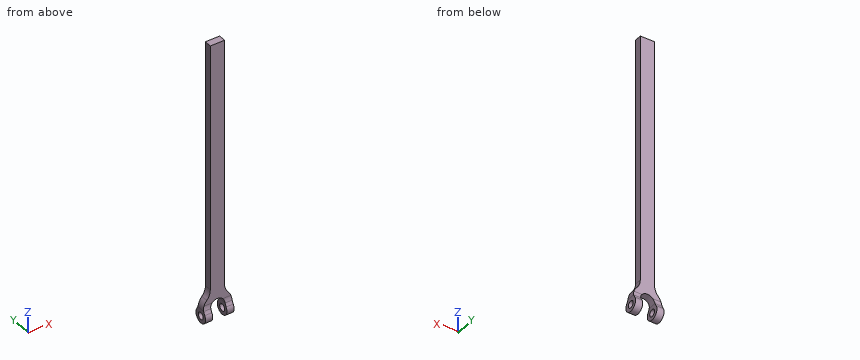
```python
from build123d import *

# Parameters (mm, degrees)
BOSS_EXTRUDE1_DEPTH = 10
CUT_EXTRUDE5_DEPTH  = 103.46950766


with BuildPart() as part:
    # Sketch1 → Boss-Extrude1 (new body)
    with BuildSketch(Plane(origin=(0, 0, 0), x_dir=(1, 0, 0), z_dir=(0, 1, 0))):
        with BuildLine():
            ThreePointArc((5, 90), (0, 85), (-5, 90))
            Line((-5, 90), (-5, 98.660254038))
            ThreePointArc((-5, 98.660254038), (-8.660254037, 95.000000002), (-10, 90.000000004))
            ThreePointArc((-10, 90.000000004), (-9.354143468, 86.464466096), (-7.5, 83.385621722))
            ThreePointArc((-7.5, 83.385621722), (-5.645856533, 80.306777351), (-5, 76.771243445))
            Line((-5, 76.771243445), (-5, -100))
            Line((-5, -100), (5, -100))
            Line((5, -100), (5, 76.771243445))
            ThreePointArc((5, 76.771243445), (5.645856533, 80.306777351), (7.5, 83.385621722))
            ThreePointArc((7.5, 83.385621722), (9.354143466, 86.464466092), (10, 89.999999995))
            ThreePointArc((10, 89.999999995), (8.660254039, 94.999999998), (5, 98.660254038))
            Line((5, 98.660254038), (5, 90))
        make_face()
        with BuildLine():
            Line((5, 100), (5, 98.660254038))
            ThreePointArc((5, 98.660254038), (8.660254039, 94.999999998), (10, 89.999999995))
            Line((10, 89.999999995), (10, 100))
            Line((10, 100), (5, 100))
        make_face()
        with BuildLine():
            ThreePointArc((-10, 90.000000004), (-8.660254037, 95.000000002), (-5, 98.660254038))
            Line((-5, 98.660254038), (-5, 100))
            Line((-5, 100), (-10, 100))
            Line((-10, 100), (-10, 90.000000004))
        make_face()
    extrude(amount=BOSS_EXTRUDE1_DEPTH)

    # Sketch2 → Cut-Extrude5 (cut, through all)
    with BuildSketch(Plane.ZY.offset(10)):
        with BuildLine():
            ThreePointArc((-92.237664695, 9.165798128), (-91.153608851, 8.540893309), (-90, 8.056259709))
            Line((-90, 8.056259709), (-90, 10))
            Line((-90, 10), (-100, 10))
            Line((-100, 10), (-100, 0))
            Line((-100, 0), (-90, 0))
            Line((-90, 0), (-90, 1.943740291))
            ThreePointArc((-90, 1.943740291), (-91.153608851, 1.459106691), (-92.237664695, 0.834201872))
            ThreePointArc((-92.237664695, 0.834201872), (-99.998436794, 5), (-92.237664695, 9.165798128))
        make_face()
        with BuildLine():
            ThreePointArc((-90, 8.056259709), (-88.378988868, 7.640045565), (-86.711266306, 7.5))
            Line((-86.711266306, 7.5), (99.557534865, 7.5))
            Line((99.557534865, 7.5), (99.557534865, 2.5))
            Line((99.557534865, 2.5), (-86.711266306, 2.5))
            ThreePointArc((-86.711266306, 2.5), (-88.378988868, 2.359954435), (-90, 1.943740291))
            Line((-90, 1.943740291), (-90, 0))
            Line((-90, 0), (-83.385621722, 0))
            Line((-83.385621722, 0), (-76.771243445, 0))
            Line((-76.771243445, 0), (100, 0))
            Line((100, 0), (100, 10))
            Line((100, 10), (-76.771243445, 10))
            Line((-76.771243445, 10), (-83.385621722, 10))
            Line((-83.385621722, 10), (-90, 10))
            Line((-90, 10), (-90, 8.056259709))
        make_face()
        with BuildLine():
            ThreePointArc((-92.5, 5), (-93.232233047, 6.767766953), (-95, 7.5))
            Line((-95, 7.5), (-95, 2.5))
            ThreePointArc((-95, 2.5), (-93.232233047, 3.232233047), (-92.5, 5))
        make_face()
        with BuildLine():
            Line((-95, 2.5), (-95, 7.5))
            ThreePointArc((-95, 7.5), (-97.5, 5), (-95, 2.5))
        make_face()
    extrude(amount=-CUT_EXTRUDE5_DEPTH, mode=Mode.SUBTRACT)


solid = part.part
```
Geometry: final body of the model. Coordinates: model frame, mm. Round coordinates to 2 decimals unless told otherwise and drop trailing zeros. Order: outer loops, then holes, each group sorted by start corner. A loop starts at its lowest first (then second) coordinate and runs counter-clockwise, first axis right, second up. Notation, with made-up numbers: M -29,-24 L 22,-24 A29 cw 22,11 Z; hole C 43.25,-19.75 d7. An arc over 180 degrees is marked long. One line per item, written item: value.
(1) Pin query (flat end, axial travel): P1, Ø10, axis at x = -3.5, z = -56.5, coming from the +Y side; P2, Ø12, axis at x = -4, z = -56, coming from the -Y side; P3, Ø1.5, axis at x = -6, y = 3, coming from the -Z side. Return the tip coordinate at first contact, or that it passes through.
Result sheet:
P1: y = 7.5
P2: y = 2.5
P3: z = -99.84
(2) Line query: probe 1 along X at (y, z) = (5.75, -45.5); probe 2 along Y at (x, z) = (0.5, 14); probe 3 along Z at (x, y) = (3, 3.75). Output: solid intervals per line, ascending. Write a range as [from, to].
Result sheet:
probe 1: [-5, 5]
probe 2: [2.5, 7.5]
probe 3: [-86, 99.56]
(3) Cut plane B-B (x = 0). Return the cut outline in (y, z).
Result sheet:
outline: M 2.5,-85 L 7.5,-85 L 7.5,99.56 L 2.5,99.56 Z
(4) Cut plane A-A (z = -18). Return the cut outline in (x, y), and give its area (3 significant figures).
Result sheet:
outline: M -5,2.5 L 5,2.5 L 5,7.5 L -5,7.5 Z
area: 50.0 mm2
